Verification items for the finished model (mm, model axes). Face numbers are marked on the shaded views. A direction names the side the tool comes from. Coordinates: 2 decimals unless noted, no trailing zeros. Order: outer loops, then holes, each group sorted by start corner. A loop starts at its lowest first (then second) coordinate and runs counter-clockwise, first axis right, second up. Notation, with made-up numbers: (-30.5, -8.75) -> (17.5, -8.75) arc R18 cw to (17.5, 25.25) -> close; hole circle Ø10 at (-3.75, 35). An arc over 180 degrees is marked (long way). Write item = value, one per line. Start each with the question number.
1. Thickness scan on line 1 along X through (y, z) = (-2.75, -8.5); line 2 along Y through (x, z) = (-8, -3.2); line 3 along X through (y, z) = (-5.5, 6). Record the ranges inside material, lowest first. Write a range as from..to.
2. Cross-section at B-B on x = -8. Record the cut outline in (y, z), plus the area to 3 significant figures.
3. Release check for a two-part mould opening along X. For the marked faces 1, 2 and 3 record: +X half, -X half, draft (parallel to the pull), parting line (faces both ways), or undercut.
4. Go/stop test with flat-tipped pins: P1, Ø9, axis at x = 44, y = 0.5, coming from the +Z side; P2, Ø9, axis at y = 1, z = 7, coming from the -X side; P3, Ø4.5, axis at y = 2, z = -9, coming from the -X side. Record where each tip stops, or that it passes through.
5. Cross-section at C-C on y = 0. Record the cut outline in (x, z).
6. Set-up check for the marked faces 4, 5, 6, 7 and 8: record each of +Z, -Z, +X, -X, +Y, -Y from which the full face is reachable in a straight line by a thin tool's end or side.
7. Cross-section at A-A on z = -12.5. Record the cut outline in (x, y), plus the area to 3 significant figures.
8. Cross-section at D-D on y = 5.5. Record the cut outline in (x, z).
from build123d import *

# Parameters (mm, degrees)
SZKIC1_W                           = 46
SZKIC1_H                           = 30
SZKIC1_R                           = 8.2
ODGI_CIE_BAZOWE1_DEPTH             = 5
ODGI_CIE_KRAW_DZI1_STRIP_W         = 21.4732
ODGI_CIE_KRAW_DZI1_STRIP_H         = 5
ODGI_CIE_KRAW_DZI1_STRIP_CUT_DEPTH = 30
ODGI_CIE_KRAW_DZI1_DEPTH           = 30
ODGI_CIE_KRAW_DZI2_STRIP_W         = 21.4732
ODGI_CIE_KRAW_DZI2_STRIP_H         = 5
ODGI_CIE_KRAW_DZI2_STRIP_CUT_DEPTH = 30
ODGI_CIE_KRAW_DZI2_DEPTH           = 30
ODGI_CIE_KRAW_DZI3_STRIP_W         = 21.4732
ODGI_CIE_KRAW_DZI3_STRIP_H         = 5
ODGI_CIE_KRAW_DZI3_STRIP_CUT_DEPTH = 30
ODGI_CIE_KRAW_DZI3_DEPTH           = 30
OD_AM_START                        = 63
OD_AM_NARO_NIK1_DEPTH              = 5
OD_AM_START_2                      = -5
OD_AM_NARO_NIK1_2_DEPTH            = 5


# Read off the part's stored shape, not the designer's step: Odłam narożnik1
# Sheet-metal steps are written as plain solids
with BuildPart() as part:
    # Szkic1 → Odgięcie bazowe1 (new body)
    with BuildSketch(Plane.XY):
        Rectangle(SZKIC1_W, SZKIC1_H)
        with Locations((-8, 0)):
            Circle(SZKIC1_R, mode=Mode.SUBTRACT)
    extrude(amount=-ODGI_CIE_BAZOWE1_DEPTH)

    # Odgięcie krawędzi1 strip (across the edge) → Odgięcie krawędzi1 strip cut (cut)
    with BuildSketch(Plane(origin=(23, 15, -5), x_dir=(-1, 0, 0), z_dir=(0, -1, 0))):
        with Locations((-5, -2.5)):
            Rectangle(ODGI_CIE_KRAW_DZI1_STRIP_W, ODGI_CIE_KRAW_DZI1_STRIP_H)
    extrude(amount=ODGI_CIE_KRAW_DZI1_STRIP_CUT_DEPTH, mode=Mode.SUBTRACT)

    # Odgięcie krawędzi1 section (across the edge) → Odgięcie krawędzi1 (add)
    with BuildSketch(Plane(origin=(23, 15, -5), x_dir=(-1, 0, 0), z_dir=(0, -1, 0))):
        with BuildLine():
            Line((0, 0.7366), (0, 15))
            Line((0, 15), (5, 15))
            Line((5, 15), (5, 0.7366))
            ThreePointArc((5, 0.7366), (5.215745145, 0.215745145), (5.7366, 0))
            Line((5.7366, 0), (5.7366, -5))
            ThreePointArc((5.7366, -5), (1.680211239, -3.319788761), (0, 0.7366))
        make_face()
    extrude(amount=ODGI_CIE_KRAW_DZI1_DEPTH)

    # Odgięcie krawędzi2 strip (across the edge) → Odgięcie krawędzi2 strip cut (cut)
    with BuildSketch(Plane(origin=(23, -15, -20), x_dir=(0, 0, 1), z_dir=(0, 1, 0))):
        with Locations((-5, -2.5)):
            Rectangle(ODGI_CIE_KRAW_DZI2_STRIP_W, ODGI_CIE_KRAW_DZI2_STRIP_H)
    extrude(amount=ODGI_CIE_KRAW_DZI2_STRIP_CUT_DEPTH, mode=Mode.SUBTRACT)

    # Odgięcie krawędzi2 section (across the edge) → Odgięcie krawędzi2 (add)
    with BuildSketch(Plane(origin=(23, -15, -20), x_dir=(0, 0, 1), z_dir=(0, 1, 0))):
        with BuildLine():
            Line((0, 0.7366), (0, 45))
            Line((0, 45), (5, 45))
            Line((5, 45), (5, 0.7366))
            ThreePointArc((5, 0.7366), (5.215745145, 0.215745145), (5.7366, 0))
            Line((5.7366, 0), (5.7366, -5))
            ThreePointArc((5.7366, -5), (1.680211239, -3.319788761), (0, 0.7366))
        make_face()
    extrude(amount=ODGI_CIE_KRAW_DZI2_DEPTH)

    # Odgięcie krawędzi3 strip (across the edge) → Odgięcie krawędzi3 strip cut (cut)
    with BuildSketch(Plane(origin=(68, -15, -15), x_dir=(-1, 0, 0), z_dir=(0, 1, 0))):
        with Locations((-5, -2.5)):
            Rectangle(ODGI_CIE_KRAW_DZI3_STRIP_W, ODGI_CIE_KRAW_DZI3_STRIP_H)
    extrude(amount=ODGI_CIE_KRAW_DZI3_STRIP_CUT_DEPTH, mode=Mode.SUBTRACT)

    # Odgięcie krawędzi3 section (across the edge) → Odgięcie krawędzi3 (add)
    with BuildSketch(Plane(origin=(68, -15, -15), x_dir=(-1, 0, 0), z_dir=(0, 1, 0))):
        with BuildLine():
            Line((0, 0.7366), (0, 35))
            Line((0, 35), (5, 35))
            Line((5, 35), (5, 0.7366))
            ThreePointArc((5, 0.7366), (5.215745145, 0.215745145), (5.7366, 0))
            Line((5.7366, 0), (5.7366, -5))
            ThreePointArc((5.7366, -5), (1.680211239, -3.319788761), (0, 0.7366))
        make_face()
    extrude(amount=ODGI_CIE_KRAW_DZI3_DEPTH)

    # Odłam narożnik1 outline → Odłam narożnik1 (cut)
    with BuildSketch(Plane.YZ.offset(OD_AM_START)):
        with BuildLine():
            Line((-15, 20), (-15, 15))
            ThreePointArc((-15, 15), (-13.535533906, 18.535533906), (-10, 20))
            Line((-10, 20), (-15, 20))
        make_face()
        with BuildLine():
            Line((15, 20), (10, 20))
            ThreePointArc((10, 20), (13.535533906, 18.535533906), (15, 15))
            Line((15, 15), (15, 20))
        make_face()
    extrude(amount=OD_AM_NARO_NIK1_DEPTH, mode=Mode.SUBTRACT)

    # Od_am naro_nik1 2 outline → Od_am naro_nik1 2 (cut)
    with BuildSketch(Plane.XY.offset(OD_AM_START_2)):
        with BuildLine():
            ThreePointArc((-18, -15), (-21.535533906, -13.535533906), (-23, -10))
            Line((-23, -10), (-23, -15))
            Line((-23, -15), (-18, -15))
        make_face()
        with BuildLine():
            ThreePointArc((-23, 10), (-21.535533906, 13.535533906), (-18, 15))
            Line((-18, 15), (-23, 15))
            Line((-23, 15), (-23, 10))
        make_face()
    extrude(amount=OD_AM_NARO_NIK1_2_DEPTH, mode=Mode.SUBTRACT)


solid = part.part
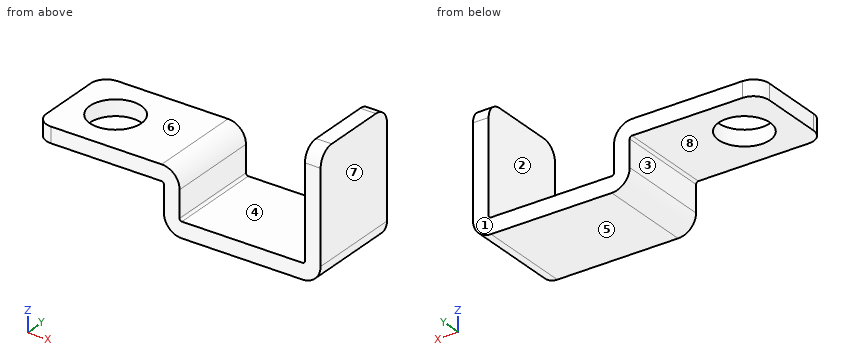
Worked out:
q1.line_1 = 18..23, 63..68
q1.line_2 = -15..-8.2, 8.2..15
q1.line_3 = 63..68
q2.outline = (-15, -5) -> (-8.2, -5) -> (-8.2, 0) -> (-15, 0) -> close; (8.2, -5) -> (15, -5) -> (15, 0) -> (8.2, 0) -> close
q2.area = 68.0 mm²
q3.face_1 = draft
q3.face_2 = undercut
q3.face_3 = -X half
q4.P1 = -15
q4.P2 = 63
q4.P3 = 18
q5.outline = (-23, -5) -> (-16.2, -5) -> (-16.2, 0) -> (-23, 0) -> close; (0.2, -5) -> (17.26, -5) arc R0.74 cw to (18, -5.74) -> (18, -14.26) arc R5.74 ccw to (23.74, -20) -> (62.26, -20) arc R5.74 ccw to (68, -14.26) -> (68, 20) -> (63, 20) -> (63, -14.26) arc R0.74 cw to (62.26, -15) -> (23.74, -15) arc R0.74 cw to (23, -14.26) -> (23, -5.74) arc R5.74 ccw to (17.26, 0) -> (0.2, 0) -> close
q6.face_4 = +Z, +Y, -Y
q6.face_5 = -Z, +X, -X, +Y, -Y
q6.face_6 = +Z, -X, +Y, -Y
q6.face_7 = +Z, -Z, +X, +Y, -Y
q6.face_8 = -Z, -X, +Y, -Y
q7.outline = (18, -15) -> (23, -15) -> (23, 15) -> (18, 15) -> close; (63, -15) -> (68, -15) -> (68, 15) -> (63, 15) -> close
q7.area = 300 mm²
q8.outline = (-23, -5) -> (-14.08, -5) -> (-14.08, 0) -> (-23, 0) -> close; (-1.92, -5) -> (17.26, -5) arc R0.74 cw to (18, -5.74) -> (18, -14.26) arc R5.74 ccw to (23.74, -20) -> (62.26, -20) arc R5.74 ccw to (68, -14.26) -> (68, 20) -> (63, 20) -> (63, -14.26) arc R0.74 cw to (62.26, -15) -> (23.74, -15) arc R0.74 cw to (23, -14.26) -> (23, -5.74) arc R5.74 ccw to (17.26, 0) -> (-1.92, 0) -> close
